Here's how the part is built. I have some questions about the finished solid (model axes, mm). Face numbers are marked on the shaded views. A direction names the side the tool comes from. Round coordinates to 2 decimals unless told otherwise and drop trailing zeros. Loops run counter-clockwise (first coordinate to the right, second up) from the corner with the lowest first, then second, coordinate; pieces in that order, holes last. Notation, with made-up numbers: M 41,24 L 84,24 A25 cw 84,63 Z; hole C -8.75,-19.75 d6. An arc over 180 degrees is marked long. Answer as a JSON object with one key per item and string values.
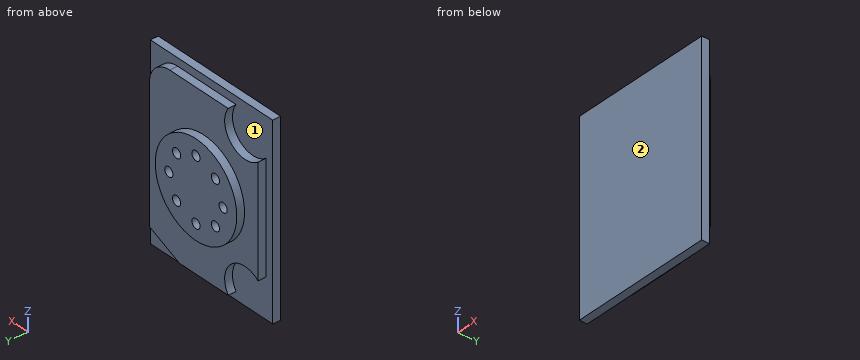
from build123d import *

# Parameters (mm, degrees)
F0_W     = 90
F0_H     = 120
F1_DEPTH = 5
F3_DEPTH = 5
F4_R     = 30
F4_R_2   = 3
F5_DEPTH = 5


with BuildPart() as f1:
    # F0 (on Front) → F1 (new body)
    with BuildSketch(Plane.XZ):
        with Locations((45, 60)):
            Rectangle(F0_W, F0_H)
    extrude(amount=F1_DEPTH)

    # F2 (on face) → F3 (join)
    with BuildSketch(Plane(origin=(0, 0, 0), x_dir=(-1, 0, 0), z_dir=(0, 1, 0))):
        with BuildLine():
            Line((-85, 15), (-63, 5))
            Line((-63, 5), (-27, 5))
            ThreePointArc((-27, 5), (-24.744746, 24.619221), (-5, 25))
            Line((-5, 25), (-5, 95))
            ThreePointArc((-5, 95), (-24.744746, 95.380779), (-27, 115))
            Line((-27, 115), (-70, 115))
            ThreePointArc((-70, 115), (-80.606602, 110.606602), (-85, 100))
            Line((-85, 100), (-85, 15))
        make_face()
    extrude(amount=F3_DEPTH)

    # F4 (on face) → F5 (join)
    with BuildSketch(Plane(origin=(0, 5, 0), x_dir=(-1, 0, 0), z_dir=(0, 1, 0))):
        with Locations((-45, 60)):
            Circle(F4_R)
        with Locations((-59.3, 46.017511)):
            Circle(F4_R_2, mode=Mode.SUBTRACT)
        with Locations((-45, 40)):
            Circle(F4_R_2, mode=Mode.SUBTRACT)
        with Locations((-30.7, 46.017511)):
            Circle(F4_R_2, mode=Mode.SUBTRACT)
        with Locations((-65, 60)):
            Circle(F4_R_2, mode=Mode.SUBTRACT)
        with Locations((-59.3, 73.982489)):
            Circle(F4_R_2, mode=Mode.SUBTRACT)
        with Locations((-45, 80)):
            Circle(F4_R_2, mode=Mode.SUBTRACT)
        with Locations((-30.7, 73.982489)):
            Circle(F4_R_2, mode=Mode.SUBTRACT)
        with Locations((-25, 60)):
            Circle(F4_R_2, mode=Mode.SUBTRACT)
    extrude(amount=F5_DEPTH)


solid = f1.part
Item 1: I want a section at A-A on z = 60. List the corners of the cut face in (x, y) for me, plus the area to 3 significant figures.
Solution:
{"outline": "M 0,-5 L 90,-5 L 90,0 L 85,0 L 85,5 L 75,5 L 75,10 L 68,10 L 68,5 L 62,5 L 62,10 L 28,10 L 28,5 L 22,5 L 22,10 L 15,10 L 15,5 L 5,5 L 5,0 L 0,0 Z", "area": "1,090 mm2"}
Item 2: If I drill on L1, parallel to Z at x = 45, y = 6.85; L2, parallel to Z at x = 31, y = 7; L3, parallel to X at y = 8.25, z = 62, over which ranges is the centre line in solid material (lowest first)? Write a range as from..to.
Solution:
{"L1": "z = 30..37, 43..77, 83..90", "L2": "z = 33.47..43.03, 49..71, 76.97..86.53", "L3": "x = 15.07..22.76, 27.24..62.76, 67.24..74.93"}
Item 3: I want a section at C-C on x = 45. List the corners of the cut face in (y, z) for me, plus the area to 3 significant figures.
Solution:
{"outline": "M -5,0 L 0,0 L 0,5 L 5,5 L 5,30 L 10,30 L 10,37 L 5,37 L 5,43 L 10,43 L 10,77 L 5,77 L 5,83 L 10,83 L 10,90 L 5,90 L 5,115 L 0,115 L 0,120 L -5,120 Z", "area": "1,390 mm2"}
Item 4: For the marked faces 1 and 2, which set-ups out of +Z, -Z, +X, -X, +Y, -Y let a thin tool reach every point of the face, with its end or its side?
Solution:
{"face 1": "+Y", "face 2": "+Z, -Z, +X, -X, -Y"}
Item 5: I want a section at B-B on y = 7. Count the separate pieces of the cut face and the enclosed holes in it, plus the area to 3 significant figures.
Solution:
{"separate pieces": "1", "enclosed holes": "8", "area": "2,600 mm2"}
Item 6: I want a section at D-D on x = 25. List the corners of the cut face in (y, z) for me.
Solution:
{"outline": "M -5,0 L 0,0 L 0,24.38 L 5,24.38 L 5,37.64 L 10,37.64 L 10,57 L 5,57 L 5,63 L 10,63 L 10,82.36 L 5,82.36 L 5,95.62 L 0,95.62 L 0,120 L -5,120 Z"}
Item 7: For P1, Ø1.5, axis at x = 36.5, y = 1.5, coming from the -Z side; P2, Ø1.5, axis at y = 1.5, z = 36, coming from the +X side; P3, Ø2.5, axis at x = 38, y = 1.5, coming from the +Z side, each with a flat end and sliding along its axis, tell me the tip position at first contact or that it passes through.
Solution:
{"P1": "stops at z = 5", "P2": "stops at x = 85", "P3": "stops at z = 115"}
